Here's how the part is built. I have some questions about the finished solid (model axes, mm). Face numbers are marked on the shaded views. A direction names the side the tool comes from. Coordinates: 2 decimals unless noted, no trailing zeros. Order: outer loops, then holes, each group sorted by start corner. A loop starts at its lowest first (then second) coordinate and runs counter-clockwise, first axis right, second up. Notation, with made-up numbers: (72, 68.5) - (89, 68.5) arc R25 ccw to (89, 88.5) - close; hole circle Ø9 at (80, -25.75). An arc over 180 degrees is marked (long way). Use one line per item in the form item = value. Start each with the question number.
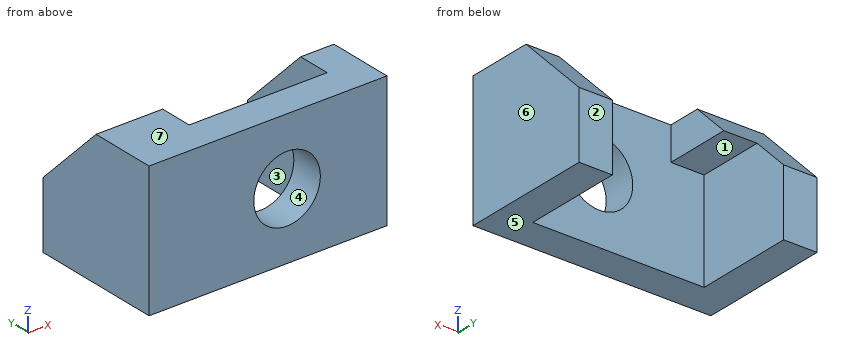
from build123d import *

# Parameters (mm, degrees)
SKETCH1_R           = 7
BOSS_EXTRUDE1_DEPTH = 7
SKETCH1_3_W         = 7
SKETCH1_3_H         = 28
BOSS_EXTRUDE2_DEPTH = 28
CHAMFER1_SIZE       = 14


with BuildPart() as part:
    # Sketch1 → Boss-Extrude1 (new body)
    with BuildSketch(Plane(origin=(0, 0, 0), x_dir=(1, 0, 0), z_dir=(0, 1, 0))):
        Polygon((18, -14), (18, 14), (-18, 14), (-18, -7), (-11, -7), (-11, -14), align=None)
        with Locations((4, 0)):
            Circle(SKETCH1_R, mode=Mode.SUBTRACT)
    extrude(amount=BOSS_EXTRUDE1_DEPTH)

    # Sketch1<3> → Boss-Extrude2 (add)
    with BuildSketch(Plane(origin=(0, 0, 0), x_dir=(1, 0, 0), z_dir=(0, 1, 0))):
        Polygon((-18, -7), (-18, 14), (-25, 14), (-25, -14), (-11, -14), (-11, -7), align=None)
        with Locations((21.5, 0)):
            Rectangle(SKETCH1_3_W, SKETCH1_3_H)
    extrude(amount=BOSS_EXTRUDE2_DEPTH)

    # Chamfer1
    chamfer1_edges = [part.edges().sort_by_distance(p)[0] for p in [
        (-18, 28, 14),
        (21.5, 28, 14),
    ]]
    chamfer(chamfer1_edges, length=CHAMFER1_SIZE)


solid = part.part
1) Suppose I cut it at B-B, the plane x = 4. List the corners of the cut face in (y, z) for me.
2) If we mould it in two halves opening along Z, with no side actions, what happens to the marked faces 4, 5, 6 and 7? For each: pulls with the +Z half, pulls with the -Z half, needs draft (parallel to the pull), parting line crosses it, or undercut.
3) I need wall thicknesses on probe 1 along X at (y, z) = (3, 0); probe 2 along X at (y, z) = (20, -12); probe 3 along Z at (x, y) = (4, 1.75). Which ranges of each line are inside material? Lowest first, please. Write a range as [from, to].
4) Suppose I cut it at D-D, the plane y = 2. List the corners of the cut face in (x, z) for me, then the cut area to 3 significant figures.
5) Suppose I cut it at C-C, the plane z = 10. List the corners of the cut face in (x, y) for me, then the cut area to 3 significant figures.
6) For pin 1 (12.5 mm diameter, centred on x = 4, z = 0, fed in from -Y); pin 2 (10 mm diameter, centred on x = 1, z = 6, fed in from +Y), each with a flat end and sliding along its axis, tell me the tip position at first contact or that it passes through.
7) Which directions (+Z, -Z, +X, -X, +Y, -Y) give clear straight access to the entire face, cutting with the end or side of a thin tool? Please do the marked faces 1, 2 and 3.
8) Suppose I cut it at A-A, the plane y = 22. List the corners of the cut face in (x, z) for me.
From the geometry:
q1.outline = (0, -14) - (7, -14) - (7, -7) - (0, -7) - close; (0, 7) - (7, 7) - (7, 14) - (0, 14) - close
q2.face_4 = undercut
q2.face_5 = pulls with the -Z half
q2.face_6 = needs draft
q2.face_7 = pulls with the +Z half
q3.probe_1 = [-25, -3], [11, 25]
q3.probe_2 = [-25, -18], [18, 25]
q3.probe_3 = [-14, -7], [7, 14]
q4.outline = (-25, -14) - (25, -14) - (25, 14) - (-25, 14) - close; hole circle Ø14 at (4, 0)
q4.area = 1,250 mm2
q5.outline = (-25, 0) - (25, 0) - (25, 18) - (18, 18) - (18, 7) - (-11, 7) - (-11, 18) - (-25, 18) - close
q5.area = 581 mm2
q6.pin_1 = through
q6.pin_2 = 7
q7.face_1 = -Z, +Y
q7.face_2 = +Z, -Z, +X, -X, +Y
q7.face_3 = +Z, -Z, +Y
q8.outline = (-25, -14) - (-18, -14) - (-18, 6) - (-25, 6) - close; (18, -14) - (25, -14) - (25, 6) - (18, 6) - close
